Read the model definition and answer for the solid it produces. Units are mm, in the model's axes. Coordinates: 2 decimals unless noted, no trailing zeros. Write each loop counter-clockwise with the first axis right and the second up, starting at its lowest first coordinate (ties: lowest second). Pieces come first, ordered by that corner, then holes. Notation, with made-up numbers: (-16, 52) -> (13, 52) arc R30 ccw to (13, 77) -> close; hole circle Ø11 at (55, -38.75). An arc over 180 degrees is marked (long way). Return JSON: item names as keys, results as strings.
Autodesk Inventor part; units mm, degrees
ref_plane "YZ Plane" through (0, 0, 0) normal (1, 0, 0) x (0, 1, 0)
ref_plane "XZ Plane" through (0, 0, 0) normal (0, 1, 0) x (-1, 0, 0)
ref_plane "XY Plane" through (0, 0, 0) normal (0, 0, 1) x (1, 0, 0)
sketch "Sketch1" plane through (0, 0, 0) normal (0, 0, 1) x (1, 0, 0)
  line L0 (0, 0) -> (304.8, 0) construction
  line L1 (304.8, 0) -> (304.8, 50.8) construction
  line L2 (304.8, 50.8) -> (0, 50.8) construction
  line L3 (0, 50.8) -> (0, 0) construction
  circle A0 centre (152.4, 23.8125) radius 6.35 construction
  circle A1 centre (152.4, 23.8125) radius 34.29 construction
  circle A2 centre (152.4, 23.8125) radius 22.225 construction
  line L4 (152.4, 23.8125) -> (139.52, 61.741) construction
  circle A3 centre (139.52, 61.741) radius 9.525 construction
  circle A4 centre (139.52, 61.741) radius 17.78 construction
  circle A5 centre (91.5619, 85.09) radius 31.75 construction
  circle A6 centre (163.3424, 109.4657) radius 31.75 construction
  line L5 (0, 50.8) -> (0, 53.34) construction
  line L6 (0, 53.34) -> (304.8, 53.34) construction
  line L7 (304.8, 53.34) -> (304.8, 50.8) construction
  circle A7 centre (139.52, 61.741) radius 21.59 construction
  circle A8 centre (152.4, 23.8125) radius 46.99 construction
  circle A9 centre (152.4, 23.8125) radius 50.8 construction
  arc A10 (86.3865, 79.4564) -> (92.4363, 92.6899) centre (91.5619, 85.09) ccw construction
  circle A11 centre (163.3424, 109.4657) radius 7.65 construction
  circle A12 centre (163.3424, 109.4657) radius 9.1 construction
  circle A13 centre (139.52, 61.741) radius 22.9 construction
  line L8 (86.3865, 79.4564) -> (124.0276, 44.8769) construction
  line L9 (170.8782, 108.1486) -> (162.078, 57.7984) construction
  line L10 (92.4363, 92.6899) -> (91.5619, 85.09) construction
  line L11 (91.5619, 85.09) -> (86.3865, 79.4564) construction
  arc A14 (128.9499, 92.8673) -> (131.407, 97.9722) centre (127.6738, 96.6252) ccw
  circle A15 centre (127.6738, 96.6252) radius 7.9375 construction
  line L12 (92.4363, 92.6899) -> (126.7664, 88.7398) construction
  line L13 (133.1953, 90.9229) -> (158.0208, 114.9615) construction
  line L14 (158.0208, 114.9615) -> (163.3424, 109.4657) construction
  line L15 (170.8782, 108.1486) -> (163.3424, 109.4657) construction
  line L16 (139.52, 61.741) -> (127.6738, 96.6252) construction
  line L17 (91.5619, 85.09) -> (163.3424, 109.4657) construction
  line L18 (152.4, 23.8125) -> (91.5619, 85.09) construction
  line L19 (152.4, 23.8125) -> (163.3424, 109.4657) construction
  circle A16 centre (127.6738, 96.6252) radius 9.2075 construction
  circle A17 centre (127.6738, 96.6252) radius 6.1595 construction
  arc A18 (92.4363, 92.6899) -> (86.3865, 79.4564) centre (91.5619, 85.09) ccw construction
  circle A19 centre (163.3424, 109.4657) radius 25.4 construction
  line L20 (104.7627, 113.9656) -> (78.361, 56.2144) construction
  circle A20 centre (91.5619, 85.09) radius 25.4 construction
  line L21 (104.4015, 107.0791) -> (92.7013, 84.5343) construction
  line L22 (81.0012, 61.9895) -> (90.3961, 85.5882) construction
  arc A21 (100.6718, 111.3992) -> (98.9102, 106.9744) centre (99.791, 109.1868) ccw construction
  arc A22 (103.3046, 104.9655) -> (105.4983, 109.1926) centre (104.4015, 107.0791) ccw construction
  arc A23 (103.3046, 104.9655) -> (98.9102, 106.9744) centre (81.0012, 61.9895) ccw construction
  line L23 (99.791, 109.1868) -> (100.6718, 111.3992) construction
  line L24 (104.4015, 107.0791) -> (105.4983, 109.1926) construction
  arc A24 (105.4983, 109.1926) -> (100.6718, 111.3992) centre (81.0012, 61.9895) ccw construction
  arc A25 (88.0213, 75.5164) -> (97.3814, 93.5522) centre (92.7013, 84.5343) ccw construction
  line L25 (90.3961, 85.5882) -> (99.791, 109.1868) construction
  line L26 (92.7013, 84.5343) -> (81.0012, 61.9895) construction
  arc A26 (88.0213, 75.5164) -> (86.6381, 76.1487) centre (81.0012, 61.9895) ccw construction
  arc A27 (97.3814, 93.5522) -> (94.1541, 95.0276) centre (81.0012, 61.9895) ccw construction
  arc A28 (94.1541, 95.0276) -> (86.6381, 76.1487) centre (90.3961, 85.5882) ccw construction
  line L27 (163.3424, 109.4657) -> (140.8985, 121.3583) construction
  line L28 (163.3424, 109.4657) -> (185.7862, 97.5731) construction
  circle A29 centre (139.52, 61.741) radius 26.71 construction
  circle A30 centre (152.4, 23.8125) radius 11.176 construction
  line L29 (152.4, 23.8125) -> (158.5256, 5.7742) construction
  circle A31 centre (152.4, 23.8125) radius 5.5065
  line L30 (156.5338, 34.1959) -> (148.2662, 13.4291) construction
  circle A32 centre (156.5338, 34.1959) radius 2.1082
  circle A33 centre (148.2662, 13.4291) radius 2.1082
  arc A34 (166.3874, 21.8643) -> (163.8992, 15.6142) centre (152.4, 23.8125) ccw
  circle A35 centre (111.304, 39.007) radius 9.525 construction
  circle A36 centre (175.745, 60.8903) radius 9.525 construction
  arc A37 (113.6108, 42.2365) -> (109.0199, 35.7614) centre (111.304, 39.007) ccw
  arc A38 (179.4939, 59.5878) -> (171.9486, 62.0473) centre (175.745, 60.8903) ccw
  arc A39 (157.2494, 9.5322) -> (156.2414, 2.5286) centre (158.5256, 5.7742) ccw
  line L31 (152.4, 23.8125) -> (165.1433, 18.7393) construction
  line L32 (166.3874, 21.8643) -> (163.8992, 15.6142)
  arc A40 (163.8992, 15.6142) -> (166.3874, 21.8643) centre (152.4, 23.8125) ccw construction
  line L33 (163.8992, 15.6142) -> (162.4566, 5.2282)
  line L34 (156.2414, 2.5286) -> (109.0199, 35.7614)
  line L35 (166.3874, 21.8643) -> (179.4939, 59.5878)
  arc A41 (123.8923, 95.4203) -> (128.9499, 92.8673) centre (127.6738, 96.6252) ccw
  arc A42 (131.407, 97.9722) -> (123.8923, 95.4203) centre (127.6738, 96.6252) ccw
  arc A43 (131.202, 98.5513) -> (131.407, 97.9722) centre (178.6686, 115.0239) ccw
  arc A44 (162.4566, 5.2282) -> (157.2494, 9.5322) centre (158.5256, 5.7742) ccw
  arc A45 (156.2414, 2.5286) -> (162.4566, 5.2282) centre (158.5256, 5.7742) ccw
  circle A46 centre (135.6607, 73.1057) radius 37.9355
  point P0 (102.1225, 108.1905)
  point P1 (145.0256, 46.8513)
  dimension "d1" = 50.8
  dimension "d3" = 23.8125
  dimension "d4" = 152.4
  dimension "d7" = 68.58
  dimension "d8" = 44.45
  dimension "d9" = 19.05
  dimension "d10" = 35.56
  dimension "d11" = 40.0558
  dimension "d12" = 63.5
  dimension "d13" = 63.5
  dimension "d15" = 2.54
  dimension "d16" = 304.8
  dimension "d17" = 43.18
  dimension "d18" = 93.98
  dimension "d19" = 101.6
  dimension "d21" = 15.3
  dimension "d22" = 15.3
  dimension "d24" = 18.2
  dimension "d29" = 45.8
  dimension "d30" = 143.991
  dimension "d31" = 7.9375
  dimension "d32" = 15.875
  dimension "d33" = 143.991
  dimension "d35" = 18.415
  dimension "d37" = 12.319
  dimension "d40" = 50.8
  dimension "d42" = 18.004
  dimension "d43" = 18.004
  dimension "d44" = 50.8
  dimension "d75" = 2.86
  dimension "d80" = 4.7625
  dimension "d82" = 4.7625
  dimension "d83" = 50.8
  dimension "d84" = 50.8
  dimension "d97" = 48.4188
  dimension "d99" = 20.32
  dimension "d101" = 25.4
  dimension "d102" = 25.4
  dimension "d103" = 10.16
  dimension "d105" = 18.004
  dimension "d106" = 18.004
  dimension "d107" = 53.42
  dimension "d149" = 22.352
  dimension "d152" = 180
  dimension "d163" = 11.013
  dimension "d190" = 12.7
  dimension "d191" = 4.2164
  dimension "d192" = 4.2164
  dimension "d209" = 28.2448
  dimension "d210" = 19.05
  dimension "d211" = 19.05
  dimension "d212" = 7.9375
  dimension "d214" = 19.05
  dimension "d215" = 7.9375
  dimension "d216" = 13.716
  dimension "d232" = 3.9688
extrude "Extrusion3" add sketch "Sketch1" along normal blind 3.175 contours L32 A34 | A34 A46 A38 L35 | A34 L33 A44 A39 L34 A37 A46 | A45 A39 A44
hole "Hole3" at (81.0012, 61.9895, 0) at (185.7862, 97.5731, 0) at (127.6738, 96.6252, 0) at (111.304, 39.007, 0) at (175.745, 60.8903, 0) at (158.5256, 5.7742, 0) direction (0, 0, 1) diameter 4.9784 end through all
fillet "Fillet3" radius 3.175 2 edges at (166.3874, 21.8643, 1.5875) (163.8992, 15.6142, 1.5875)
equation "\"d8\" = Gear35tPD"
equation "\"d9\" = Gear15tPD"
equation "\"d10\" = Gear28tPD"
equation "\"d11\" = 0.5 * Gear48tPD + 0.5 * Gear15tPD + MeshingClearance"
equation "\"d12\" = CimOD"
equation "\"d13\" = CimOD"
equation "\"d17\" = Gear28tPD + ClearanceDiameter"
equation "\"d18\" = WheelOD"
equation "\"d19\" = WheelClearance"
equation "\"Pulley48tPD\" = 45.8"
equation "\"Pulley19tPD\" = 18.2"
equation "\"Pulley16tPD\" = 15.3"
equation "\"Gear15tPD\" = 19.05"
equation "\"Gear35tPD\" = 44.45"
equation "\"Gear48tPD\" = 60.96"
equation "\"Gear28tPD\" = 35.56"
equation "\"BearingLargeOD\" = 28.575"
equation "\"BearingSmallOD\" = 22.225"
equation "\"MeshingClearance\" = 0.0508"
equation "\"CimOD\" = 63.5"
equation "\"WheelOD\" = 93.98"
equation "\"ClearanceDiameter\" = 7.62"
equation "\"WheelClearance\" = 101.6"
equation "\"TensioningBearingID\" = 6.35"
equation "\"TensioningBearingOD\" = 15.875"
equation "\"SpingClipClearance\" = 8.89"
equation "\"Pi\" = 79.79645"
equation "\"Pulley56tPD\" = 53.5"
equation "\"BearingXLargeOD\" = 34.925"
properties part number "OutlineSketch1" material "Aluminum 6061"
1. The part is cut by section B-B (z = 1.15). Count the separate pieces of the cut face and the enclosed holes in it, then the cut area to 3 significant figures.
Taken from the geometry:
{"separate pieces": "1", "enclosed holes": "6", "area": "1,350 mm2"}
2. The part is cut by section A-A (x = 152.4). Determine the outline of the cut face in (y, z) (3 decimals).
Taken from the geometry:
{"outline": "(5.232, 0) -> (18.306, 0) -> (18.306, 3.175) -> (5.232, 3.175) -> close; (29.319, 0) -> (39.063, 0) -> (39.063, 3.175) -> (29.319, 3.175) -> close"}
3. For a pull along X with two mould halves and no side action, classify faces 1 (the face through (176.89, 64.69, 1.57)), 2 (the face through (177.26, 58.915, 1.61)), 3 (the face through (149, 29, 0)) as +X half, -X half, draft (parallel to the pull), parting line (faces both ways), or undercut.
Taken from the geometry:
{"face 1": "parting line", "face 2": "undercut", "face 3": "draft"}
4. Consider L1, parallel to X at y = 41, z = 0.4; L2, parallel to Y at x = 156, z = 2; L3, parallel to Y at x = 148, z = 1.35. Determine where each line is inside the solid, lowest interval first.
Taken from the geometry:
{"L1": "x = 107.87 to 109.81, 112.8 to 115.45, 155.87 to 173.04", "L2": "y = 2.7 to 19.65, 27.98 to 32.16, 36.24 to 41.08", "L3": "y = 8.33 to 11.34, 15.52 to 20.5, 27.12 to 37.23"}
5. The part is cut by section D-D (y = 45.5). Determine the outline of the cut face in (x, z) (3 decimals).
Taken from the geometry:
{"outline": "(161.68, 0) -> (174.599, 0) -> (174.599, 3.175) -> (161.68, 3.175) -> close"}
6. Flat-ended cylindrical pins translate along their axes: pin 1 Ø10 at (x, y) = (160, 53.5) entering from +Z; pin 2 Ø1 at (y, z) = (12, 2.5) entering from -X. Find the tip coordinate at first contact, or state that the pin passes through.
Taken from the geometry:
{"pin 1": "passes through", "pin 2": "stops at x = 142.07"}
7. The part is cut by section C-C (x = 115). Determine the outline of the cut face in (y, z) (3 decimals), then the cut area to 3 significant figures.
Taken from the geometry:
{"outline": "(31.553, 0) -> (41.29, 0) -> (41.29, 3.175) -> (31.553, 3.175) -> close", "area": "30.9 mm2"}
